Source: CAD feature listing. Evaluate the final solid. Frame: model axes, mm. Round coordinates to 2 decimals unless told otherwise and drop trailing zeros. Loops run counter-clockwise (first coordinate to the right, second up) from the corner with the lowest first, then second, coordinate; pieces in that order, holes last. Notation, with made-up numbers: M -17,75 L 12,75 A19 ccw 12,110 Z; hole C -32,43.5 d5. An arc over 180 degrees is marked long. Answer as a JSON object with one key per item and string values.
Autodesk Inventor part; units mm, degrees
ref_plane "YZ Plane" through (0, 0, 0) normal (1, 0, 0) x (0, 1, 0)
ref_plane "XZ Plane" through (0, 0, 0) normal (0, 1, 0) x (-1, 0, 0)
ref_plane "XY Plane" through (0, 0, 0) normal (0, 0, 1) x (1, 0, 0)
sketch "Sketch1" plane through (0, 0, 0) normal (0, 0, 1) x (1, 0, 0)
  line L0 (0, 0) -> (190.5, 0)
  line L1 (190.5, 0) -> (190.5, 635)
  line L2 (190.5, 635) -> (0, 635)
  line L3 (0, 635) -> (0, 0)
  dimension "d0" = 190.5
  dimension "d1" = 635
extrude "Extrusion1" add sketch "Sketch1" along normal blind 3.175
sketch "Sketch2" plane through (0, 0, 3.175) normal (0, 0, 1) x (1, 0, 0)
  line L0 (0, 0) -> (0, 635)
  line L1 (190.5, 0) -> (0, 0)
  line L2 (165.1, 0) -> (0, 0)
  line L3 (0, 177.8) -> (165.1, 0)
  line L4 (0, 635) -> (190.5, 635)
  line L5 (165.1, 635) -> (0, 635)
  line L6 (0, 533.4) -> (165.1, 635)
  line L7 (0, 533.4) -> (0, 635)
  line L8 (165.1, 635) -> (165.1, 0) construction
  line L9 (190.5, 635) -> (190.5, 0)
  dimension "d5" = 177.8
  dimension "d8" = 101.6
  dimension "d9" = 25.4
extrude "Extrusion2" cut sketch "Sketch2" against normal up to next contours L0 L3 L1 | L0 L4 L6
sketch "Sketch4" plane through (0, 0, 3.175) normal (0, 0, 1) x (1, 0, 0)
  line L0 (0, 177.8) -> (0, 533.4)
  line L1 (0, 444.5) -> (50.8, 444.5)
  line L2 (50.8, 444.5) -> (50.8, 368.3)
  line L3 (50.8, 368.3) -> (0, 368.3)
  line L4 (0, 368.3) -> (0, 444.5)
  line L5 (165.1, 635) -> (50.8, 635) construction
  line L6 (50.8, 635) -> (50.8, 444.5) construction
  line L7 (50.8, 368.3) -> (50.8, 0) construction
  line L8 (50.8, 0) -> (165.1, 0) construction
  point P0 (0, 0)
  dimension "d17" = 76.2
  dimension "d18" = 50.8
  dimension "d27" = 190.5
extrude "ConveyorHole" cut sketch "Sketch4" against normal through all
properties part number "Conveyor_Frame_BottomStabilizerPlate" material "Aluminum-6061"
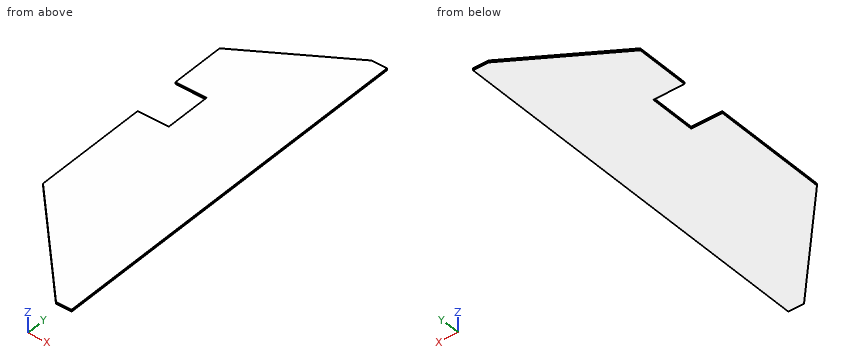
Item 1: Section D-D on y = 146.5. Return the cut outline in (x, z) (3 decimals).
Answer sheet:
{"outline": "M 29.064,0 L 190.5,0 L 190.5,3.175 L 29.064,3.175 Z"}
Item 2: Section A-A on x = 13.5. Return the cut outline in (y, z) (3 decimals), then the cut area to 3 significant figures.
Answer sheet:
{"outline": "M 163.262,0 L 368.3,0 L 368.3,3.175 L 163.262,3.175 Z; M 444.5,0 L 541.708,0 L 541.708,3.175 L 444.5,3.175 Z", "area": "960 mm²"}
Item 3: Section C-C on x = 97.5. Return the cut outline in (y, z) (3 decimals), then the cut area to 3 significant figures.
Answer sheet:
{"outline": "M 72.8,0 L 593.4,0 L 593.4,3.175 L 72.8,3.175 Z", "area": "1,650 mm²"}
Item 4: Section B-B on z = 2.5. Return the cut outline in (x, y), then the cut area to 3 significant figures.
Answer sheet:
{"outline": "M 0,177.8 L 165.1,0 L 190.5,0 L 190.5,635 L 165.1,635 L 0,533.4 L 0,444.5 L 50.8,444.5 L 50.8,368.3 L 0,368.3 Z", "area": "94,000 mm²"}
Item 5: Line query: probe 1 along Y at (x, z) = (8, 2.7); probe 2 along Y at (x, z) = (32.5, 0.45); probe 3 along X at (y, z) = (173, 2.7). Output: solid intervals per line, ascending. Write a range as from..to.
Answer sheet:
{"probe 1": "y = 169.18..368.3, 444.5..538.32", "probe 2": "y = 142.8..368.3, 444.5..553.4", "probe 3": "x = 4.46..190.5"}
Item 6: Contact query for a flat-ended pin moving along its axis: pin 1 Ø1.5 at (x, z) = (25.5, 2.5) entering from -Y. Output: stop coordinate, or through.
Answer sheet:
{"pin 1": "stops at y = 149.53"}
